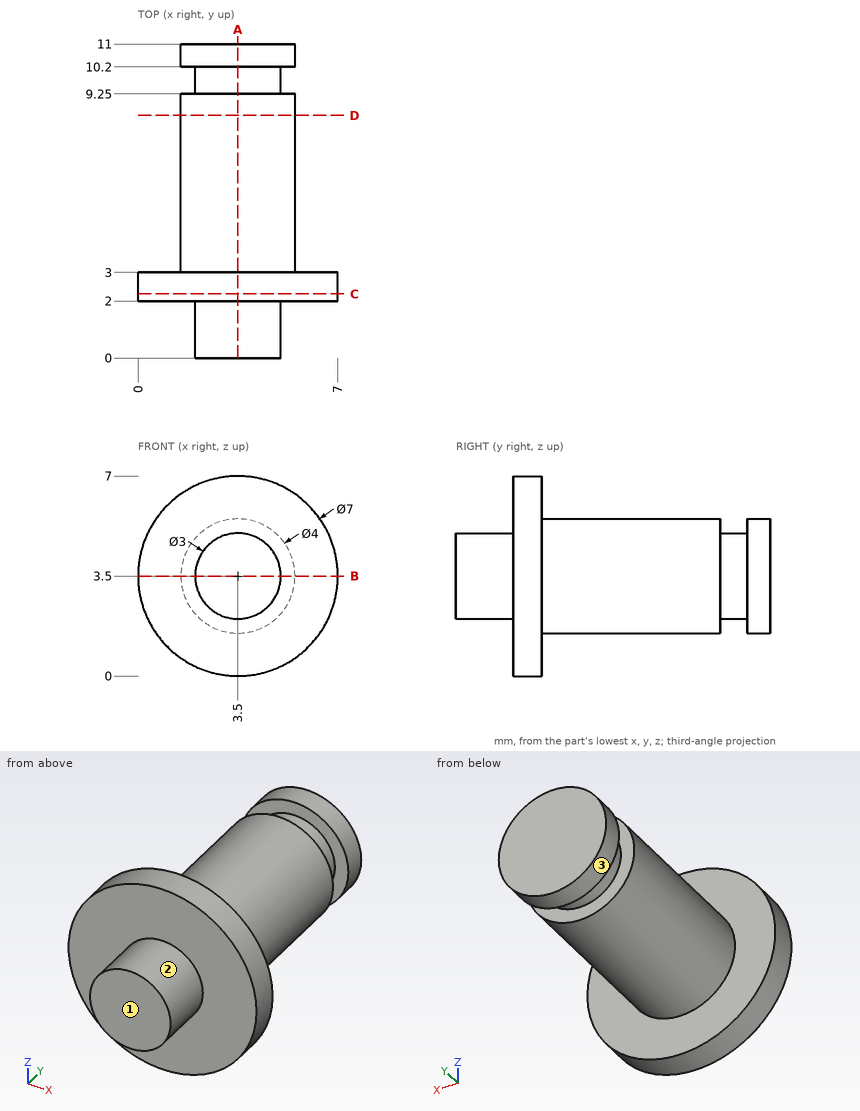
Geometry: see drawing. Coordinates: mm, zero at the bounding-box minimum. A direction names the side the tool comes from. Coordinates: 2 decimals unless noted, no trailing zeros. Loops run counter-clockwise (first coordinate to the right, second up) from the corner with the lowest first, then second, coordinate; pieces in that order, holes last. Notation, with made-up numbers: (-30.75, 41.25) - (14.25, 41.25) arc R7 cw to (14.25, 47.25) - close; hole circle Ø8 at (20, 31.25). An arc over 180 degrees is marked (long way). Answer as CSV lines item,"result".
1. Reachability of the marked faces 1, 2 and 3 from +Z, -Z, +X, -X, +Y, -Y: full face, straight path, thin tool, end or side. Return the list, or none.
Established:
face 1,"+Z, -Z, +X, -X, -Y"
face 2,"-Y"
face 3,"+Y"
2. Section C-C (y = 2.25). Return loops of the section in (x, z).
Established:
outline,"circle Ø7 at (3.5, 3.5)"
3. Section B-B (z = 3.5). Return loops of the section in (x, y).
Established:
outline,"(0, 2) - (2, 2) - (2, 0) - (5, 0) - (5, 2) - (7, 2) - (7, 3) - (5.5, 3) - (5.5, 9.25) - (5, 9.25) - (5, 10.2) - (5.5, 10.2) - (5.5, 11) - (1.5, 11) - (1.5, 10.2) - (2, 10.2) - (2, 9.25) - (1.5, 9.25) - (1.5, 3) - (0, 3) - close"
4. Contact query for flat-ended pins moving along their axis: pin 1 (1.5 mm diameter, centred on y = 7, z = 5, fed in from -X); pin 2 (2 mm diameter, centred on x = 1, y = 8, fed in from +Z). Output: stop coordinate, or through.
Established:
pin 1,"stops at x = 1.65"
pin 2,"stops at z = 4.82"
5. Section D-D (y = 8.5). Return loops of the section in (x, z).
Established:
outline,"circle Ø4 at (3.5, 3.5)"
6. Ray query, line 1 (Y direction, x = 1.75, z = 4); line 2 (Y direction, x = 1, z = 5); line 3 (Z direction, x = 1.75, y = 4.25). Return the intervals inside material, ascending.
Established:
line 1,"y = 2 to 9.25, 10.2 to 11"
line 2,"y = 2 to 3"
line 3,"z = 2.53 to 4.47"
7. Section A-A (x = 3.5). Return loops of the section in (y, z), then the cut area to 4 significant figures.
Established:
outline,"(0, 2) - (2, 2) - (2, 0) - (3, 0) - (3, 1.5) - (9.25, 1.5) - (9.25, 2) - (10.2, 2) - (10.2, 1.5) - (11, 1.5) - (11, 5.5) - (10.2, 5.5) - (10.2, 5) - (9.25, 5) - (9.25, 5.5) - (3, 5.5) - (3, 7) - (2, 7) - (2, 5) - (0, 5) - close"
area,"44.05 mm2"
